```python
from build123d import *

# Parameters (mm, degrees)
F0_W          = 8.5162539035
F0_H          = 18.7663150777
F0_H_2        = 40.954434668
F1_DEPTH      = 8
F2_R          = 3
F3_R          = 1.5
F4_DEPTH      = 25
F5_R          = 2
F6_DEPTH      = 13.4
F6_DEPTH_BACK = 25
F7_SIZE       = 1
F8_R          = 6.5791532239
F9_DEPTH      = 25
F10_R         = 1


with BuildPart() as f1:
    # F0 (on Top) → F1 (new body)
    with BuildSketch(Plane.XY):
        Polygon((11.7504801601, 36.198887974), (11.7504801601, 59.4197693529), (4.2642612243, 59.4197693529), (4.2642612243, 40.6534542753), (-4.2519926792, 40.6534542753), (-4.2519926792, 59.4197693529), (-11.7504801601, 59.4197693529), (-11.7504801601, 36.198887974), align=None)
        with Locations((0.0061342726, 50.0366118141)):
            Rectangle(F0_W, F0_H)
        with Locations((0.0061342726, 79.8969866869)):
            Rectangle(F0_W, F0_H_2)
    extrude(amount=-F1_DEPTH)

    # F2
    f2_edges = [f1.edges().sort_by_distance(p)[0] for p in [
        (-11.75048, 59.419769, -4),
        (11.75048, 59.419769, -4),
        (-4.251993, 100.374204, -4),
        (4.264261, 100.374204, -4),
        (0, 36.198888, -8),
        (-8.001236, 59.419769, -8),
        (8.007371, 59.419769, -8),
        (-11.75048, 47.809329, -8),
        (11.75048, 47.809329, -8),
        (0.006134, 100.374204, -8),
    ]]
    fillet(f2_edges, radius=F2_R)

    # F3 (on Top) → F4 (cut)
    with BuildSketch(Plane.XY):
        with Locations((-6.6438065842, 43.8586436212)):
            Circle(F3_R)
        with Locations((6.6438065842, 43.8586436212)):
            Circle(F3_R)
    extrude(amount=-F4_DEPTH, mode=Mode.SUBTRACT)

    # F5 (on Right) → F6 (cut, two sides)
    with BuildSketch(Plane.YZ) as f6_sk:
        with Locations((88.9796987176, -4.4162971899)):
            Circle(F5_R)
    extrude(amount=-F6_DEPTH, mode=Mode.SUBTRACT)
    extrude(f6_sk.sketch, amount=F6_DEPTH_BACK, mode=Mode.SUBTRACT)

    # F7
    f7_edges = [f1.edges().sort_by_distance(p)[0] for p in [
        (4.264261, 86.979699, -4.416297),
        (-4.251993, 86.979699, -4.416297),
    ]]
    chamfer(f7_edges, length=F7_SIZE)

    # F8 (on Top) → F9 (cut)
    with BuildSketch(Plane.XY):
        with Locations((8.0665275455, 68.2693198323)):
            Circle(F8_R)
        with Locations((-8.0665275455, 68.2693198323)):
            Circle(F8_R)
    extrude(amount=-F9_DEPTH, mode=Mode.SUBTRACT)

    # F10
    f10_edges = [f1.edges().sort_by_distance(p)[0] for p in [
        (-1.487374, 68.26932, -8),
        (1.487374, 68.26932, -8),
        (4.264261, 62.900146, -4),
        (4.264261, 73.638494, -4),
        (-4.251993, 62.908855, -4),
        (-4.251993, 73.629784, -4),
    ]]
    fillet(f10_edges, radius=F10_R)


solid = f1.part
```
Geometry: final body of the model. Coordinates: model frame, mm. A direction names the side the tool comes from. Round coordinates to 2 decimals unless told otherwise and drop trailing zeros. Order: outer loops, then holes, each group sorted by start corner. A loop starts at its lowest first (then second) coordinate and runs counter-clockwise, first axis right, second up. Notation, with made-up numbers: M 69.25,-38 L 116.25,-38 A15 ccw 116.25,-27 Z; hole C 18,-13.75 d2. An arc over 180 degrees is marked long. Use one line per item in the form item = value. Start each with the question number.
Q1. Cut plane C-C (y = 47.5). Return loops of the section in (x, z), and give its area (3 significant figures).
Q2. Cut plane D-D (z = -3.5). Count the separate pieces of the cut face and the enclosed holes in it, and give its area (3 significant figures).
Q3. Cut plane B-B (z = -0.75). Return loops of the section in (x, y).
Q4. Cut plane A-A (x = 6.25). Return loops of the section in (y, z), and give its area (3 significant figures).
Q5. Pin query (flat end, axial travel): pin 1 Ø2 at (x, z) = (7.5, -5.5) entering from -Y; pin 2 Ø4 at (y, z) = (62.5, -2) entering from -X; pin 3 Ø8 at (x, y) = (8.5, 82) entering from +Z; pin 4 Ø3 at (x, z) = (-4, -1.5) entering from +Y. Return the tip coordinate at first contact, or that it passes through.
Q6. Access query for faces 1 (the face through (0.165, 37.054, -7.098)), 2 (the face through (-6, 59.42, -2)), 3 (the face through (6.48, 58.56, -7.1)), 4 (the face through (0.07, 99.12, -7.44)), 5 (the face through (7, 59.42, -2)). Directions: +Z, -Z, +X, -X, +Y, -Y. A direction counts if a zero-diameter tool reaches every point of the face in a straight line with its end or side. Return the directions, or none.
Q7. Material intervals for line 1 (Y direction, x = 2.5, z = -4); line 2 (Y direction, x = -2, z = -4.25); line 3 (X direction, y = 84.5, z = -5.75), sorted ascending. Write a range as [from, to].
Q8. Mould query, pull axis Z, two halves, no side actions, for faces 6 (the face through (-6.53, 58.56, -7.1)), 7 (the face through (0, 100.374, -2)), 8 (the face through (0, 62, 0)). Classes: +Z half, -Z half, draft (parallel to the pull), parting line (faces both ways), or undercut.
Geometry results:
q1.outline = M -11.75,-5 A3 ccw -8.75,-8 L 8.75,-8 A3 ccw 11.75,-5 L 11.75,0 L -11.75,0 Z
q1.area = 184 mm^2
q2.separate_pieces = 2
q2.enclosed_holes = 2
q2.area = 798 mm^2
q3.outline = M -11.75,36.2 L 11.75,36.2 L 11.75,56.42 A3 ccw 8.75,59.42 L 4.26,59.42 L 4.26,62.41 A1 ccw 3.9,63.18 A6.58 cw 3.9,73.36 A1 ccw 4.26,74.13 L 4.26,97.37 A3 ccw 1.26,100.37 L -1.25,100.37 A3 ccw -4.25,97.37 L -4.25,74.12 A1 ccw -3.89,73.35 A6.58 cw -3.89,63.19 A1 ccw -4.25,62.42 L -4.25,59.42 L -8.75,59.42 A3 ccw -11.75,56.42 Z; hole C -6.64,43.86 d3; hole C 6.64,43.86 d3
q4.outline = M 36.2,-5 A3 ccw 39.2,-8 L 42.41,-8 L 42.41,0 L 36.2,0 Z; M 45.31,-8 L 56.42,-8 A3 ccw 59.42,-5 L 59.42,0 L 45.31,0 Z
q4.area = 159 mm^2
q5.pin_1 = 36.2
q5.pin_2 = -4.25
q5.pin_3 = through
q5.pin_4 = 100.1
q6.face_1 = -Z, +X, -X, -Y
q6.face_2 = +Z, -Z, -X, +Y
q6.face_3 = -Z, +X, +Y
q6.face_4 = -Z, +X, -X, +Y
q6.face_5 = +Z, -Z, +X, +Y
q7.line_1 = [36.2, 64.76], [71.78, 87.02], [90.94, 100.11]
q7.line_2 = [36.2, 65.72], [70.82, 86.99], [90.97, 100.28]
q7.line_3 = [-4.25, 4.26]
q8.face_6 = -Z half
q8.face_7 = draft
q8.face_8 = +Z half
